Answer from the drawing. Dimensions are ordinates in mm from the lowest x, y and z of the part. A direction names the side the tool comes from. Give positions to 0.01 mm unless a question says otherwise; leave off trailing zeros. Loops run counter-clockwise (first coordinate to the right, second up) from the corner with the lowest first, then second, coordinate; pieces in that order, holes last. Notation, with made-up numbers: (38, 39) - (56, 39) arc R20 cw to (56, 48) - close; hole circle Ø10 at (62.25, 46.25). An arc over 180 degrees is marked (long way). Put each result on its own line as item: value. Start each with the question number.
1. A cutting plane is placed at A-A, the plane x = 15. Determine the outline of the cut face in (y, z), plus the area to 3 significant figures.
2. Given pin 1 Ø5.5 at (y, z) = (18, 12) entering from -X; pin 2 Ø1 at (y, z) = (11.5, 4) entering from +X; pin 3 Ø9.5 at (x, z) = (102.5, 8.5) entering from -Y, each flat-ended and moving along its own axis, determine where each tip first touches the part or whether it passes through.
3. A cutting plane is placed at C-C, the plane y = 30. Determine the outline of the cut face in (x, z), plus the area to 3 significant figures.
4. A cutting plane is placed at D-D, the plane x = 136.5. Determine the outline of the cut face in (y, z).
5. For a pull along Z with two mould halves and no side action, classify the marked faces 1, 2, 3 and 4 as released by +Z, released by -Z, zero draft, split by the parting line, or undercut.
6. A cutting plane is placed at B-B, the plane z = 19.5. Determine the outline of the cut face in (x, y) (3 decimals).
7. Consider L1, parallel to Z at x = 9.5, y = 26; L2, parallel to Y at x = 124.5, z = 14; L3, parallel to X at y = 35.5, z = 25.5. Determine where each line is inside the solid, lowest interval first. Write a range as from..to.
8. For the marked faces 5, 6 and 7, determine the directions among +Z, -Z, +X, -X, +Y, -Y from which every point of the face is accessible in a straight line to the end or side of a thin tool.
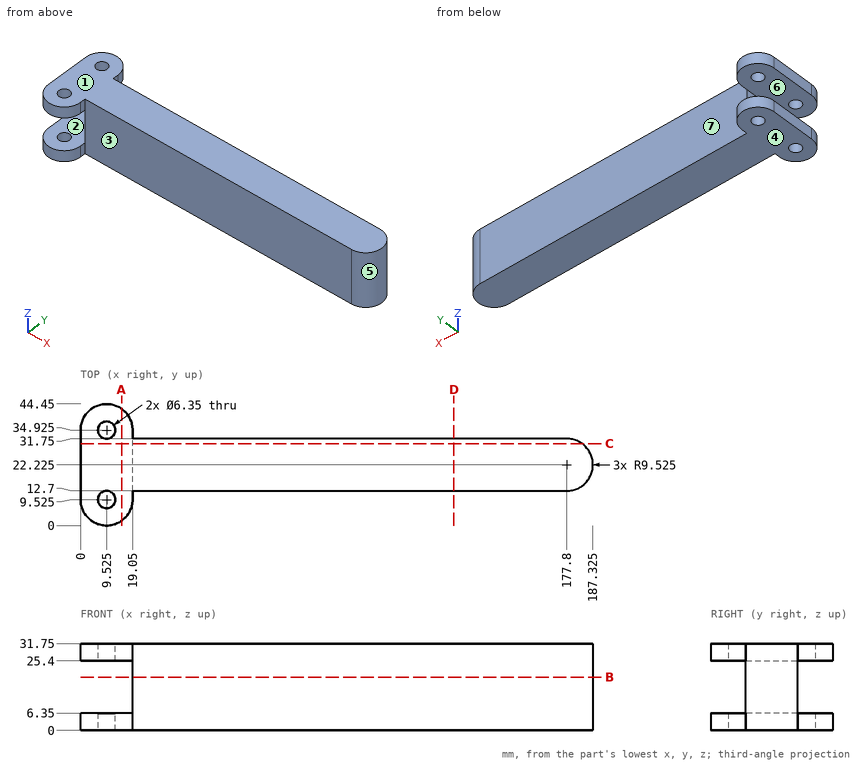
Return value:
1. outline: (1.73, 0) - (42.72, 0) - (42.72, 6.35) - (1.73, 6.35) - close; (1.73, 25.4) - (42.72, 25.4) - (42.72, 31.75) - (1.73, 31.75) - close
1. area: 521 mm2
2. pin 1: stops at x = 19.05
2. pin 2: stops at x = 19.05
2. pin 3: stops at y = 12.7
3. outline: (0, 0) - (183.3, 0) - (183.3, 31.75) - (0, 31.75) - (0, 25.4) - (19.05, 25.4) - (19.05, 6.35) - (0, 6.35) - close
3. area: 5,460 mm2
4. outline: (12.7, 0) - (31.75, 0) - (31.75, 31.75) - (12.7, 31.75) - close
5. face 1: released by +Z
5. face 2: undercut
5. face 3: zero draft
5. face 4: released by -Z
6. outline: (19.05, 12.7) - (177.8, 12.7) arc R9.525 ccw to (177.8, 31.75) - (19.05, 31.75) - close
7. L1: z = 0..6.35, 25.4..31.75
7. L2: y = 12.7..31.75
7. L3: x = 0.02..6.4, 12.65..19.03
8. face 5: +Z, -Z, +X
8. face 6: -X, +Y, -Y
8. face 7: +Z, -Z, +X, +Y
